Model file for the job. Use its own axes, mm. A direction names the side the tool comes from. Give positions to 0.01 mm unless a question says otherwise; leave off trailing zeros. Order: outer loops, then holes, each group sorted by start corner. A loop starts at its lowest first (then second) coordinate and runs counter-clockwise, first axis right, second up. Notation, with made-up numbers: M 24.5,27 L 31.5,27 A15 cw 31.5,44 Z; hole C 28.5,-34.75 d7. An arc over 180 degrees is marked long. Return JSON: item names as keys, results as strings. Group by question number.
1. Pin check, flat tips, straight feed: pin 1 (6 mm diameter, centred on x = 21.1, z = -6.28, fed in from +Y); pin 2 (4 mm diameter, centred on y = -5, z = 27, fed in from +X); pin 3 (6.5 mm diameter, centred on x = 46, y = -6, fed in from +Z) (3 decimals); pin 4 (6.5 mm diameter, centred on y = -7, z = 20, fed in from -X). Stop position of each tip, or through.
2. Slice it at A-A on x = 34. List the corners of the cut face in (y, z).
3. Slice it at B-B on z = -5. Give the number of separate pieces and of enclosed holes in the cut face, then the cut area to 3 significant figures.
4. 3-axis set-ups, long thin cutter, end or side, ignore diameter. For faces 5 (the face through (51.944, -6.261, -5.484)), 6 (the face through (-4.151, -6, 23)), 7 (the face through (21.249, -6, 22)): which of +Z, -Z, +X, -X, +Y, -Y reach the whole face in a straight line?
5. Two-plate mould, pull along Z, no slides. Class faces 1 (the face through (11.1, -6.26, 22.84)), 2 (the face through (59.349, -6, -6)), 3 (the face through (-23, -6, 3.705)), 4 (the face through (8, -6, -15.345)): released by +Z, released by -Z, zero draft, split by the parting line, or undercut.
6. Wall check: probe 1 along X at (y, z) = (-9.75, 23.5); probe 2 along Z at (x, y) = (7, -4.75); probe 3 along Z at (x, y) = (-15.5, -2.5). Give the ranges that are in metal, low to high. Write a range as [from, to].
7. Slice it at D-D on x = 48.5. List the corners of the cut face in (y, z), then the cut area to 3 significant figures.
from build123d import *

# Parameters (mm, degrees)
F0_R     = 2.404306
F0_R_2   = 2.684776
F0_R_3   = 2.53436
F0_R_4   = 2.677502
F0_R_5   = 2.694859
F0_R_6   = 2.671458
F0_R_7   = 2.644601
F0_R_8   = 2.644603
F0_R_9   = 2.672879
F0_R_10  = 2.225712
F1_DEPTH = 12.7


with BuildPart() as f1:
    # F0 (on Front) → F1 (new body)
    with BuildSketch(Plane.XZ):
        Polygon((-42.251352, -15.345026), (59.348648, -15.345026), (59.348648, 3.704974), (21.248648, 3.704974), (21.248648, 41.804974), (-4.151352, 41.804974), (-4.151352, 3.704974), (-42.251352, 3.704974), align=None)
        with Locations((-32.591719, -6.277913)):
            Circle(F0_R, mode=Mode.SUBTRACT)
        with Locations((-18.700166, -6.277913)):
            Circle(F0_R_2, mode=Mode.SUBTRACT)
        with Locations((-4.808613, -6.277913)):
            Circle(F0_R_3, mode=Mode.SUBTRACT)
        with Locations((8.548648, -6.277913)):
            Circle(F0_R_4, mode=Mode.SUBTRACT)
        with Locations((8.548648, 9.750801)):
            Circle(F0_R_5, mode=Mode.SUBTRACT)
        with Locations((21.104472, -6.277913)):
            Circle(F0_R_6, mode=Mode.SUBTRACT)
        with Locations((35.26317, -6.277913)):
            Circle(F0_R_7, mode=Mode.SUBTRACT)
        with Locations((49.421869, -6.277913)):
            Circle(F0_R_8, mode=Mode.SUBTRACT)
        with Locations((8.548648, 22.039484)):
            Circle(F0_R_9, mode=Mode.SUBTRACT)
        with Locations((8.548648, 32.458149)):
            Circle(F0_R_10, mode=Mode.SUBTRACT)
    extrude(amount=F1_DEPTH)


solid = f1.part
Result:
{
 "1": {"pin 1": "stops at y = 0", "pin 2": "stops at x = 21.25", "pin 3": "stops at z = 3.705", "pin 4": "stops at x = -4.15"},
 "2": {"outline": "M -12.7,-15.35 L 0,-15.35 L 0,-8.6 L -12.7,-8.6 Z; M -12.7,-3.95 L 0,-3.95 L 0,3.7 L -12.7,3.7 Z"},
 "3": {"separate pieces": "8", "enclosed holes": "0", "area": "886 mm2"},
 "4": {"face 5": "+Y, -Y", "face 6": "+Z, -X, +Y, -Y", "face 7": "+Z, +X, +Y, -Y"},
 "5": {"face 1": "undercut", "face 2": "zero draft", "face 3": "released by +Z", "face 4": "released by -Z"},
 "6": {"probe 1": "x = [-4.15, 6.31], [10.79, 21.25]", "probe 2": "z = [-15.35, -8.46], [-4.09, 7.55], [11.96, 19.86], [24.22, 30.86], [34.06, 41.8]", "probe 3": "z = [-15.35, 3.7]"},
 "7": {"outline": "M -12.7,-15.35 L 0,-15.35 L 0,-8.76 L -12.7,-8.76 Z; M -12.7,-3.8 L 0,-3.8 L 0,3.7 L -12.7,3.7 Z", "area": "179 mm2"}
}
